Source: CAD feature listing. Evaluate the final solid. Frame: model axes, mm. Give positions to 0.01 mm unless a question says otherwise; leave off trailing zeros. Write each loop counter-clockwise with the first axis right and the second up, starting at its lowest first coordinate (ties: lowest second). Pieces come first, ordered by that corner, then holes. Notation, with made-up numbers: (-39, -7) -> (-35, -7) arc R9 ccw to (-35, 10) -> close; hole circle Ø7 at (60, 6). An arc over 180 degrees is marked (long way). Answer as a JSON object with one key per item and string values. Group by question number.
Item 1: Ray query, probe 1 along X at (y, z) = (7, 0.6); probe 2 along X at (y, z) = (-12.5, 0.9); probe 3 along Y at (x, z) = (-40.5, 0.7). Return the intervals inside material, ascending. Write a range as from..to.
Item 2: Section query C-C on x = 150.5. Return the cut outline in (y, z), plus the area to 3 significant figures.
Item 3: Section query A-A on z = 1.75. Give the number of separate pieces and of enclosed holes in the cut face, plus the area to 3 significant figures.
Item 4: Section query B-B on y = 73.5. Return the cut outline in (x, z).
Item 5: First-contact query: pin 1 Ø1.3 at (x, z) = (126.5, 1.5) entering from -Y; pin 2 Ø1.3 at (x, z) = (197.5, 1.5) entering from +Y. Flat tips, straight axial feed; report the tip coordinate or a pass-through.
from build123d import *

# Parameters (mm, degrees)
F1_DEPTH = 2.54
F2_W     = 4.0894
F2_H     = 5.08
F3_DEPTH = 25.4
F4_DEPTH = 25.4


with BuildPart() as f1:
    # F0 (on Top) → F1 (new body)
    with BuildSketch(Plane.XY):
        with BuildLine():
            Line((126.392629, 190.480612), (-126.392629, 190.480612))
            ThreePointArc((-126.392629, 190.480612), (0, -228.6), (126.392629, 190.480612))
        make_face()
    extrude(amount=F1_DEPTH)

    # F2 (on face) → F3 (cut)
    with BuildSketch(Plane.XY.offset(2.54)):
        with Locations((-197.973407, 0)):
            Rectangle(F2_W, F2_H)
        with Locations((-126.363405, 0)):
            Rectangle(F2_W, F2_H)
        with Locations((-197.973407, 50.8)):
            Rectangle(F2_W, F2_H)
        with Locations((-197.973407, -50.8)):
            Rectangle(F2_W, F2_H)
        with Locations((-126.363405, 101.6)):
            Rectangle(F2_W, F2_H)
        with Locations((-126.363405, -101.6)):
            Rectangle(F2_W, F2_H)
        with Locations((197.973407, 0)):
            Rectangle(F2_W, F2_H)
        with Locations((197.973407, -50.8)):
            Rectangle(F2_W, F2_H)
        with Locations((197.973407, 50.8)):
            Rectangle(F2_W, F2_H)
        with Locations((126.363405, 0)):
            Rectangle(F2_W, F2_H)
        with Locations((126.363405, -101.6)):
            Rectangle(F2_W, F2_H)
        with Locations((126.363405, 101.6)):
            Rectangle(F2_W, F2_H)
    extrude(amount=-F3_DEPTH, mode=Mode.SUBTRACT)

    # F2 (on face) → F4 (cut)
    with BuildSketch(Plane.XY.offset(2.54)):
        with Locations((126.363405, 101.6)):
            Rectangle(F2_W, F2_H)
        with Locations((197.973407, 50.8)):
            Rectangle(F2_W, F2_H)
        with Locations((126.363405, 0)):
            Rectangle(F2_W, F2_H)
        with Locations((197.973407, 0)):
            Rectangle(F2_W, F2_H)
        with Locations((197.973407, -50.8)):
            Rectangle(F2_W, F2_H)
        with Locations((126.363405, -101.6)):
            Rectangle(F2_W, F2_H)
    extrude(amount=-F4_DEPTH, mode=Mode.SUBTRACT)


solid = f1.part
Worked answers:
{
 "1": {"probe 1": "-228.49..228.49", "probe 2": "-228.26..228.26", "probe 3": "-224.98..190.48"},
 "2": {"outline": "(-172.07, 0) -> (172.07, 0) -> (172.07, 2.54) -> (-172.07, 2.54) -> close", "area": "874 mm^2"},
 "3": {"separate pieces": "1", "enclosed holes": "12", "area": "157,000 mm^2"},
 "4": {"outline": "(-216.46, 0) -> (216.46, 0) -> (216.46, 2.54) -> (-216.46, 2.54) -> close"},
 "5": {"pin 1": "y = -190.84", "pin 2": "y = 116.22"}
}
